Read the model definition and answer for the solid it produces. Units are mm, in the model's axes. A direction names the side the tool comes from. Give positions to 0.01 mm unless a question says otherwise; leave off trailing zeros. Order: outer loops, then holes, each group sorted by start corner. A loop starts at its lowest first (then second) coordinate and runs counter-clockwise, first axis right, second up.
Autodesk Inventor part; units mm, degrees
ref_plane "YZ Plane" through (0, 0, 0) normal (1, 0, 0) x (0, 1, 0)
ref_plane "XZ Plane" through (0, 0, 0) normal (0, 1, 0) x (-1, 0, 0)
ref_plane "XY Plane" through (0, 0, 0) normal (0, 0, 1) x (1, 0, 0)
sketch "Sketch1" plane through (0, 0, 0) normal (1, 0, 0) x (0, 1, 0)
  circle A0 centre (0, 0) radius 10
  circle A1 centre (-379, 0) radius 10
  line L0 (0, 0) -> (-379, 0) construction
  line L1 (20, 22.5) -> (-399, 22.5)
  line L2 (-399, 22.5) -> (-399, -22.5)
  line L3 (-399, -22.5) -> (20, -22.5)
  line L4 (20, -22.5) -> (20, 22.5)
  line L5 (20, 0) -> (-399, 0) construction
  dimension "d0" = 20
  dimension "d2" = 20
  dimension "d3" = 379
  dimension "d4" = 45
  dimension "d5" = 20
extrude "Extrusion1" add sketch "Sketch1" along normal mid plane 24
sketch "Sketch2" plane through (12, 0, 0) normal (1, 0, 0) x (0, 0, -1)
  circle A0 centre (0, 0) radius 10
  line L0 (22.5, -399) -> (22.5, 20)
  line L1 (22.5, 20) -> (-22.5, 20)
  line L2 (-22.5, 20) -> (22.5, 20)
  line L3 (22.5, 20) -> (22.5, -89)
  line L4 (22.5, -89) -> (-22.5, -89)
  line L5 (-22.5, -89) -> (-22.5, 20)
  circle A1 centre (0, 0) radius 10
  dimension "d8" = 109
extrude "Extrusion2" add sketch "Sketch2" along normal blind 25
mirror "Mirror1" about plane through (0, 0, 0) normal (1, 0, 0) of "Extrusion2"
sketch "Sketch3" plane through (-12, -399, 22.5) normal (0, 0, 1) x (1, 0, 0)
  line L0 (49, 419) -> (-25, 419)
  line L1 (-15, 419) -> (39, 419)
  line L2 (39, 419) -> (39, 320)
  line L3 (39, 320) -> (-15, 320)
  line L4 (-15, 320) -> (-15, 419)
  line L5 (12, 419) -> (12, 320) construction
  point P0 (12, 399)
  dimension "d11" = 99
  dimension "d13" = 54
extrude "Extrusion3" cut sketch "Sketch3" against normal through all
move or copy body "Move Body1" bodies to move or copy 1 copy no rotation origin (0, 0, 0) rotation axis (1, 0, 0) rotation angle 90
move or copy body "Move Body2" bodies to move or copy 1 copy no rotation origin (0, 0, 0) rotation axis (0, 0, 1) rotation angle 90
properties part number "UpperLeg_v2"
1) Consider L1, parallel to Y at x = 9, z = -52; L2, parallel to Z at x = 0, y = 32.75; L3, parallel to Z at x = 18.5, y = 2.5. Determine where each line is inside the solid, lowest interval first.
Final values:
L1: y = -37 to -27, 27 to 37
L2: z = -89 to -10, 10 to 20
L3: z = -399 to -79
2) The part is cut by section C-C on z = 0. Determine the outline of the cut face in (x, y).
Final values:
outline: (-22.5, -37) - (-10, -37) - (-10, -27) - (-22.5, -27) - close; (-22.5, 27) - (-10, 27) - (-10, 37) - (-22.5, 37) - close; (10, -37) - (22.5, -37) - (22.5, -27) - (10, -27) - close; (10, 27) - (22.5, 27) - (22.5, 37) - (10, 37) - close
3) The part is cut by section A-A on z = -379. Determine the outline of the cut face in (x, y), and give its area (3 significant figures).
Final values:
outline: (-22.5, -12) - (-10, -12) - (-10, 12) - (-22.5, 12) - close; (10, -12) - (22.5, -12) - (22.5, 12) - (10, 12) - close
area: 600 mm2
4) The part is cut by section D-D on y = 6.5. Determine the outline of the cut face in (x, z).
Final values:
outline: (-22.5, -399) - (22.5, -399) - (22.5, -79) - (-22.5, -79) - close; hole circle Ø20 at (0, -379)
5) The part is cut by section B-B on x = 6. Determine the outline of the cut face in (y, z), and give its area (3 significant figures).
Final values:
outline: (-37, -89) - (-12, -89) - (-12, -371) - (12, -371) - (12, -89) - (37, -89) - (37, -8) - (27, -8) - (27, -79) - (-27, -79) - (-27, -8) - (-37, -8) - close; (-37, 8) - (-27, 8) - (-27, 20) - (-37, 20) - close; (-12, -399) - (12, -399) - (12, -387) - (-12, -387) - close; (27, 8) - (37, 8) - (37, 20) - (27, 20) - close
area: 9,460 mm2
6) A tool of negligible diameter and unlimited length cuts with its end or side. For faces 1 (the face through (0, 32, 20)), 2 (the face through (0, 0, -79)), 3 (the face through (0, 24, -89)), 4 (the face through (2.17, 31.93, 9.76)), 5 (the face through (0, -12, -246)), from which of +Z, -Z, +X, -X, +Y, -Y can it reach the whole face along a straight path? Write none if from no direction.
Final values:
face 1: +Z, +X, -X, +Y, -Y
face 2: +Z, +X, -X
face 3: -Z, +X, -X, +Y
face 4: +Y, -Y
face 5: -Z, +X, -X, -Y
7) Given pin 1 (16 mm diameter, centred on x = 0, z = -379, fed in from -Y); pin 2 (1 mm diameter, centred on x = 9.5, z = -348, fed in from +Y); pin 3 (7.5 mm diameter, centred on x = -3.5, y = -18.5, fed in from -Z); pin 4 (2 mm diameter, centred on x = 18, z = -340.5, fed in from -Y), each flat-ended and moving along its own axis, determine where each tip first touches the part or whether it passes through.
Final values:
pin 1: passes through
pin 2: stops at y = 12
pin 3: stops at z = -89
pin 4: stops at y = -12
8) For a pull along X with two mould halves and no side action, classify faces 6 (the face through (0, -24, -89)), 7 (the face through (-22.5, 3, -189)), 8 (the face through (2.17, -31.93, -9.76)) as released by +X, released by -X, zero draft, split by the parting line, or undercut.
Final values:
face 6: zero draft
face 7: released by -X
face 8: undercut
